```python
from build123d import *

# Parameters (mm, degrees)
SKETCH1_W                                       = 125
SKETCH1_H                                       = 125
SKETCH1_R                                       = 3.724428854
BOSS_EXTRUDE2_DEPTH                             = 6
SKETCH3_R                                       = 2
CUT_EXTRUDE1_DEPTH                              = 5
CSK_FOR_M5_FLAT_HEAD_MACHINE_SCREW1_D           = 5.8
CSK_FOR_M5_FLAT_HEAD_MACHINE_SCREW1_DEPTH       = 6
CSK_FOR_M5_FLAT_HEAD_MACHINE_SCREW1_CSINK_D     = 10.4
CSK_FOR_M5_FLAT_HEAD_MACHINE_SCREW1_CSINK_ANGLE = 90
CSK_FOR_M5_FLAT_HEAD_MACHINE_SCREW1_TIP         = 1.742495795
CSK_FOR_M5_FLAT_HEAD_MACHINE_SCREW3_D           = 5.8
CSK_FOR_M5_FLAT_HEAD_MACHINE_SCREW3_DEPTH       = 6
CSK_FOR_M5_FLAT_HEAD_MACHINE_SCREW3_CSINK_D     = 10.4
CSK_FOR_M5_FLAT_HEAD_MACHINE_SCREW3_CSINK_ANGLE = 90
CSK_FOR_M5_FLAT_HEAD_MACHINE_SCREW3_TIP         = 1.742495795
CSK_FOR_M5_FLAT_HEAD_MACHINE_SCREW4_D           = 5.8
CSK_FOR_M5_FLAT_HEAD_MACHINE_SCREW4_DEPTH       = 6
CSK_FOR_M5_FLAT_HEAD_MACHINE_SCREW4_CSINK_D     = 10.4
CSK_FOR_M5_FLAT_HEAD_MACHINE_SCREW4_CSINK_ANGLE = 90
CSK_FOR_M5_FLAT_HEAD_MACHINE_SCREW4_TIP         = 1.742495795
CSK_FOR_M5_FLAT_HEAD_MACHINE_SCREW5_D           = 5.8
CSK_FOR_M5_FLAT_HEAD_MACHINE_SCREW5_DEPTH       = 6
CSK_FOR_M5_FLAT_HEAD_MACHINE_SCREW5_CSINK_D     = 10.4
CSK_FOR_M5_FLAT_HEAD_MACHINE_SCREW5_CSINK_ANGLE = 90
CSK_FOR_M5_FLAT_HEAD_MACHINE_SCREW5_TIP         = 1.742495795


with BuildPart() as part:
    # Sketch1 → Boss-Extrude2 (new body)
    with BuildSketch(Plane(origin=(0, 0, 0), x_dir=(1, 0, 0), z_dir=(0, 1, 0))):
        Rectangle(SKETCH1_W, SKETCH1_H)
        with Locations(Location((50, 30, 0), (0, 0, 270))):
            Circle(SKETCH1_R, mode=Mode.SUBTRACT)
        with Locations(Location((-50, 30, 0), (0, 0, 270))):
            Circle(SKETCH1_R, mode=Mode.SUBTRACT)
        with Locations(Location((-50, -30, 0), (0, 0, 270))):
            Circle(SKETCH1_R, mode=Mode.SUBTRACT)
        with Locations(Location((50, -30, 0), (0, 0, 270))):
            Circle(SKETCH1_R, mode=Mode.SUBTRACT)
    extrude(amount=BOSS_EXTRUDE2_DEPTH)

    # Sketch3 → Cut-Extrude1 (cut)
    with BuildSketch(Plane(origin=(0, 0, -62.5), x_dir=(-1, 0, 0), z_dir=(0, 0, -1))):
        with Locations((0.738370199, 3)):
            Circle(SKETCH3_R)
    extrude(amount=-CUT_EXTRUDE1_DEPTH, mode=Mode.SUBTRACT)

    # CSK for M5 Flat Head Machine Screw1
    with Locations(Plane(origin=(50, 0, -30), x_dir=(0, 0, -1), z_dir=(0, -1, 0))):
        with Locations((0, 0)):
            CounterSinkHole(CSK_FOR_M5_FLAT_HEAD_MACHINE_SCREW1_D / 2, CSK_FOR_M5_FLAT_HEAD_MACHINE_SCREW1_CSINK_D / 2, depth=CSK_FOR_M5_FLAT_HEAD_MACHINE_SCREW1_DEPTH, counter_sink_angle=CSK_FOR_M5_FLAT_HEAD_MACHINE_SCREW1_CSINK_ANGLE)
            with Locations((0, 0, -(CSK_FOR_M5_FLAT_HEAD_MACHINE_SCREW1_DEPTH + CSK_FOR_M5_FLAT_HEAD_MACHINE_SCREW1_TIP / 2))):  # 118° drill point
                Cone(0, CSK_FOR_M5_FLAT_HEAD_MACHINE_SCREW1_D / 2, CSK_FOR_M5_FLAT_HEAD_MACHINE_SCREW1_TIP, mode=Mode.SUBTRACT)

    # CSK for M5 Flat Head Machine Screw3
    with Locations(Plane(origin=(-50, 0, -30), x_dir=(0, 0, -1), z_dir=(0, -1, 0))):
        with Locations((0, 0)):
            CounterSinkHole(CSK_FOR_M5_FLAT_HEAD_MACHINE_SCREW3_D / 2, CSK_FOR_M5_FLAT_HEAD_MACHINE_SCREW3_CSINK_D / 2, depth=CSK_FOR_M5_FLAT_HEAD_MACHINE_SCREW3_DEPTH, counter_sink_angle=CSK_FOR_M5_FLAT_HEAD_MACHINE_SCREW3_CSINK_ANGLE)
            with Locations((0, 0, -(CSK_FOR_M5_FLAT_HEAD_MACHINE_SCREW3_DEPTH + CSK_FOR_M5_FLAT_HEAD_MACHINE_SCREW3_TIP / 2))):  # 118° drill point
                Cone(0, CSK_FOR_M5_FLAT_HEAD_MACHINE_SCREW3_D / 2, CSK_FOR_M5_FLAT_HEAD_MACHINE_SCREW3_TIP, mode=Mode.SUBTRACT)

    # CSK for M5 Flat Head Machine Screw4
    with Locations(Plane(origin=(-50, 0, 30), x_dir=(0, 0, -1), z_dir=(0, -1, 0))):
        with Locations((0, 0)):
            CounterSinkHole(CSK_FOR_M5_FLAT_HEAD_MACHINE_SCREW4_D / 2, CSK_FOR_M5_FLAT_HEAD_MACHINE_SCREW4_CSINK_D / 2, depth=CSK_FOR_M5_FLAT_HEAD_MACHINE_SCREW4_DEPTH, counter_sink_angle=CSK_FOR_M5_FLAT_HEAD_MACHINE_SCREW4_CSINK_ANGLE)
            with Locations((0, 0, -(CSK_FOR_M5_FLAT_HEAD_MACHINE_SCREW4_DEPTH + CSK_FOR_M5_FLAT_HEAD_MACHINE_SCREW4_TIP / 2))):  # 118° drill point
                Cone(0, CSK_FOR_M5_FLAT_HEAD_MACHINE_SCREW4_D / 2, CSK_FOR_M5_FLAT_HEAD_MACHINE_SCREW4_TIP, mode=Mode.SUBTRACT)

    # CSK for M5 Flat Head Machine Screw5
    with Locations(Plane(origin=(50, 0, 30), x_dir=(0, 0, -1), z_dir=(0, -1, 0))):
        with Locations((0, 0)):
            CounterSinkHole(CSK_FOR_M5_FLAT_HEAD_MACHINE_SCREW5_D / 2, CSK_FOR_M5_FLAT_HEAD_MACHINE_SCREW5_CSINK_D / 2, depth=CSK_FOR_M5_FLAT_HEAD_MACHINE_SCREW5_DEPTH, counter_sink_angle=CSK_FOR_M5_FLAT_HEAD_MACHINE_SCREW5_CSINK_ANGLE)
            with Locations((0, 0, -(CSK_FOR_M5_FLAT_HEAD_MACHINE_SCREW5_DEPTH + CSK_FOR_M5_FLAT_HEAD_MACHINE_SCREW5_TIP / 2))):  # 118° drill point
                Cone(0, CSK_FOR_M5_FLAT_HEAD_MACHINE_SCREW5_D / 2, CSK_FOR_M5_FLAT_HEAD_MACHINE_SCREW5_TIP, mode=Mode.SUBTRACT)


solid = part.part
```
The model under review builds one solid part; all positions refer to its coordinate system, in mm. A direction names the side the tool comes from. Coordinates: 2 decimals unless noted, no trailing zeros. Order: outer loops, then holes, each group sorted by start corner. A loop starts at its lowest first (then second) coordinate and runs counter-clockwise, first axis right, second up. Notation, with made-up numbers: M 51.5,-6 L 57.5,-6 A15 cw 57.5,0 Z; hole C 32.5,-20.5 d10. An arc over 180 degrees is marked long. One line per question, with ' | ' between items.
(1) For probe 1 along X at (y, z) = (4.3, -30); probe 2 along X at (y, z) = (4.25, -33); probe 3 along Z at (x, y) = (0, 1.9), list the stretches that pass through material, from the lowest coordinate up. Write a range as from..to.
Geometry results:
probe 1: x = -62.5..-53.72, -46.28..46.28, 53.72..62.5 | probe 2: x = -62.5..-52.21, -47.79..47.79, 52.21..62.5 | probe 3: z = -57.5..62.5
(2) Machinability: for faces 1 (the face through (-62.5, 3, 1)), 2 (the face through (-1, 3, -57.5)), which of the approach directions +Z, -Z, +X, -X, +Y, -Y give a long, thin tool a straight path to every point of the face, cutting with its end or side? Answer none if there is none.
Geometry results:
face 1: +Z, -Z, -X, +Y, -Y | face 2: -Z
(3) Add section A-A, the plane x = 50. Write out the cut boundary in (y, z), then the cut area to 3 significant figures.
Geometry results:
outline: M 0,-62.5 L 6,-62.5 L 6,-33.72 L 1.48,-33.72 L 0,-35.2 Z; M 0,-24.8 L 1.48,-26.28 L 6,-26.28 L 6,26.28 L 1.48,26.28 L 0,24.8 Z; M 0,35.2 L 1.48,33.72 L 6,33.72 L 6,62.5 L 0,62.5 Z | area: 656 mm²
(4) Insertion check: pin 1 (6 mm diameter, centred on x = 50, z = -30, fed in from +Y); pin 2 (1.2 mm diameter, centred on x = -1, y = 3.5, fed in from -Z). Each pin has a flat end and moves straight along its axis. Give the tip position at first contact, or say it passes through.
Geometry results:
pin 1: passes through | pin 2: stops at z = -57.5
(5) Add section B-B, the plane z = -30. Write out the cut boundary in (x, y), then the cut area to 3 significant figures.
Geometry results:
outline: M -62.5,0 L -55.2,0 L -53.72,1.48 L -53.72,6 L -62.5,6 Z; M -46.28,1.48 L -44.8,0 L 44.8,0 L 46.28,1.48 L 46.28,6 L -46.28,6 Z; M 53.72,1.48 L 55.2,0 L 62.5,0 L 62.5,6 L 53.72,6 Z | area: 656 mm²
(6) The part is to be moulded in two halves that separate along Z. For faces 3 (the face through (-0.3, 1.05, -60.04)), 4 (the face through (53.14, 3.71, -28)), 5 (the face through (-0.9, 0.3, -62.5)), say which applies: +Z half, -Z half, draft (parallel to the pull), parting line (faces both ways), or undercut.
Geometry results:
face 3: draft | face 4: undercut | face 5: -Z half
